Could you check a few things on this drawing? It's one solid part, dimensions in mm from its lowest x, y, z. A direction names the side the tool comes from. Give positions to 0.01 mm unless a question says otherwise; leave off trailing zeros. Order: outer loops, then holes, each group sorted by start corner. A loop starts at its lowest first (then second) coordinate and runs counter-clockwise, first axis right, second up. Notation, with made-up numbers: (87.5, -15.75) - (116.5, -15.75) arc R16 cw to (116.5, 12.25) - close; hole circle Ø11 at (9, 41.25). An arc over 180 degrees is marked (long way). Answer as CSV lines item,"result".
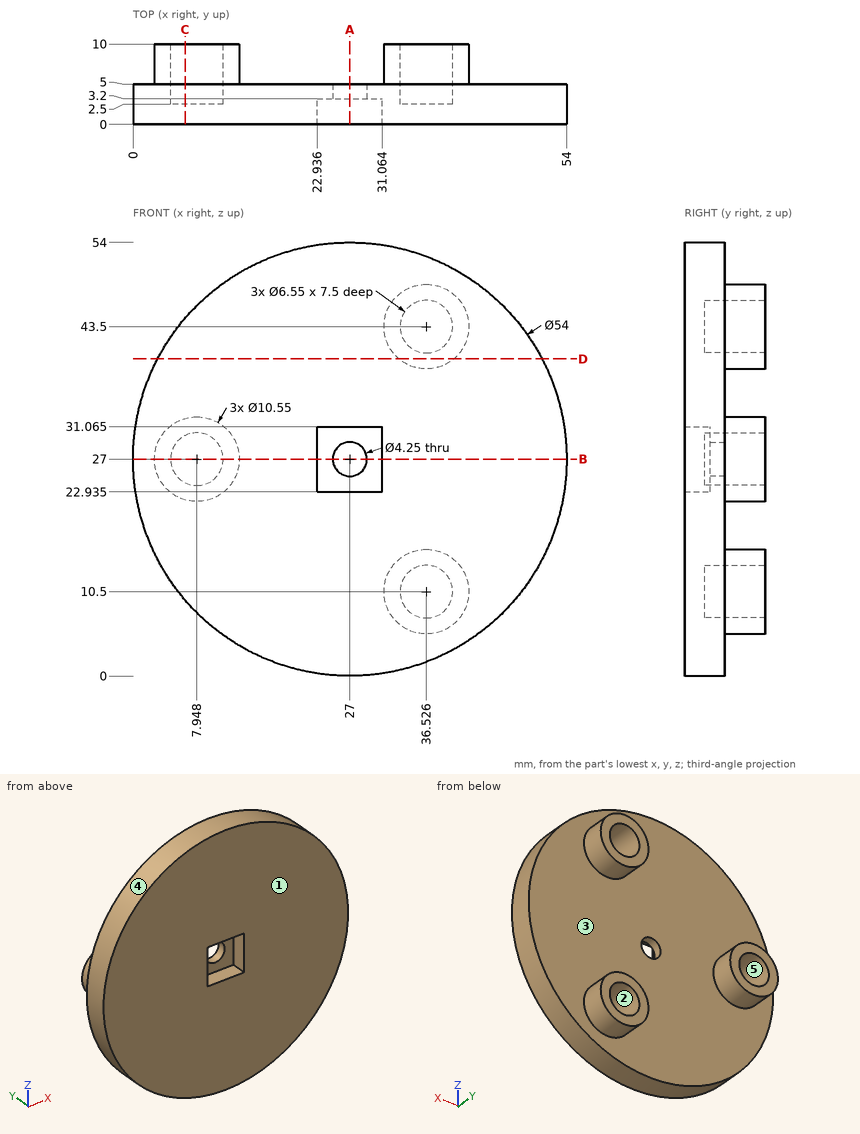
1) I need wall thicknesses on line 1 along X through (y, z) = (7.25, 27); line 2 along Z through (x, y) = (39, 5.75) (1 decimal); line 3 along Y through (x, z) = (15, 37). Which ranges of each line are inside material? Lowest first, please. Write a range as [from, to].
Answer block:
line 1,"[2.67, 4.67], [11.22, 13.22]"
line 2,"[5.8, 8.4], [12.6, 15.2], [38.8, 41.4], [45.6, 48.2]"
line 3,"[0, 5]"
2) Which directions (+Z, -Z, +X, -X, +Y, -Y) give clear straight access to the entire face, cutting with the end or side of a thin tool? Please do the marked faces 1 and 2.
Answer block:
face 1,"+Z, -Z, +X, -X, -Y"
face 2,"+Y"
3) I want a section at B-B on z = 27. Write out the boundary of the cut face in (x, y) (1 decimal), plus the area to 3 significant figures.
Answer block:
outline,"(0, 0) - (22.9, 0) - (22.9, 3.2) - (24.9, 3.2) - (24.9, 5) - (13.2, 5) - (13.2, 10) - (11.2, 10) - (11.2, 2.5) - (4.7, 2.5) - (4.7, 10) - (2.7, 10) - (2.7, 5) - (0, 5) - close; (29.1, 3.2) - (31.1, 3.2) - (31.1, 0) - (54, 0) - (54, 5) - (29.1, 5) - close"
area,"240 mm2"
4) I want a section at D-D on z = 39.5. Write out the boundary of the cut face in (x, y) (1 decimal).
Answer block:
outline,"(3.1, 0) - (50.9, 0) - (50.9, 5) - (40, 5) - (40, 10) - (33.1, 10) - (33.1, 5) - (3.1, 5) - close"
5) I want a section at C-C on x = 6.5. Write out the boundary of the cut face in (y, z), plus the area to 3 significant figures.
Answer block:
outline,"(0, 9.43) - (5, 9.43) - (5, 21.93) - (10, 21.93) - (10, 24.06) - (2.5, 24.06) - (2.5, 29.94) - (10, 29.94) - (10, 32.07) - (5, 32.07) - (5, 44.57) - (0, 44.57) - close"
area,"182 mm2"
6) I want a section at A-A on x = 27. Write out the boundary of the cut face in (y, z) (1 decimal).
Answer block:
outline,"(0, 0) - (5, 0) - (5, 24.9) - (3.2, 24.9) - (3.2, 22.9) - (0, 22.9) - close; (0, 31.1) - (3.2, 31.1) - (3.2, 29.1) - (5, 29.1) - (5, 54) - (0, 54) - close"
7) I'm going to push flat-ended pins straight in: P1, Ø3.5, axis at x = 8, z = 27, coming from the +Y side; P2, Ø5, axis at x = 37.5, z = 44.5, coming from the +Y side; P3, Ø6, axis at y = 5.5, z = 32, coming from the -X side; P4, Ø6, axis at x = 35.5, y = 4, coming from the -Z side. Where does each tip first touch, or does it pass through?
Answer block:
P1,"y = 2.5"
P2,"y = 10"
P3,"x = 0.08"
P4,"z = 0.57"
8) If we mould it in two halves opening along X, with no side actions, what happens to the marked faces 3, 4 and 5? For each: +X half, -X half, draft (parallel to the pull), parting line (faces both ways), or undercut.
Answer block:
face 3,"draft"
face 4,"parting line"
face 5,"undercut"
